```python
from build123d import *

# Parameters (mm, degrees)
PAD_DEPTH    = 9
SKETCH001_R  = 7
POCKET_DEPTH = 9
FILLET_R     = 50


with BuildPart() as part:
    # Sketch → Pad (new body)
    with BuildSketch(Plane.XY):
        Polygon((0, 94.860678), (0, 0), (0, -94.860678), (427.593604, -1000), (900, -1000), (900, 1000), (427.593604, 1000), align=None)
    extrude(amount=PAD_DEPTH)

    # Sketch001 (on DatumPlane) → Pocket (cut)
    with BuildSketch(Plane.XY.offset(9)):
        with Locations((328.804653, -388.309992)):
            Circle(SKETCH001_R)
        with Locations((116.672619, -176.177958)):
            Circle(SKETCH001_R)
    pocket = extrude(amount=-POCKET_DEPTH, mode=Mode.SUBTRACT)

    # Mirrored: Pocket across Sketch001 H_Axis
    add(pocket.mirror(Plane(origin=(0, 0, 9), x_dir=(0, 0, 1), z_dir=(0, 1, 0))), mode=Mode.SUBTRACT)

    # Fillet
    fillet_edges = [part.edges().sort_by_distance(p)[0] for p in [
        (0, 94.860678, 4.5),
        (0, -94.860678, 4.5),
        (427.593604, -1000, 4.5),
        (900, -1000, 4.5),
        (900, 1000, 4.5),
        (427.593604, 1000, 4.5),
    ]]
    fillet(fillet_edges, radius=FILLET_R)


with BuildPart() as part_1:
    # Fillet001Body placement: moved
    add(part.part.moved(Location((0, 0, 8))))


solid = part_1.part
```
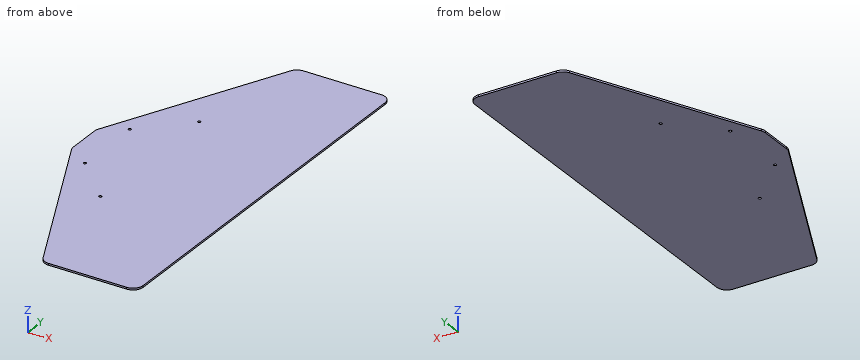
Could you check a few things on this model? Use its own coordinates, in mm. Round coordinates to 2 decimals unless told otherwise and drop trailing zeros. Loops run counter-clockwise (first coordinate to the right, second up) from the corner with the lowest first, then second, coordinate; pieces in that order, holes last. Notation, with made-up numbers: (28, 71) - (45, 71) arc R19 ccw to (45, 85) - close; hole circle Ø11 at (83.25, 12). An arc over 180 degrees is marked (long way). Answer in a Markdown table with one row per item. Add a question column.
(1) If we section it at C-C (y = 329.5): Please give me the cut outline in (x, z).
(2) I need wall thicknesses on line 1 along Y through (x, z) = (150, 15.25); line 2 along X through (y, z) = (-422, 9.75); line 3 along Y through (x, z) = (369, 15). Which ranges of each line are inside material? Lowest first, please.
(3) If we section it at B-B (x = 300): Please give me the cut outline in (y, z), plus the area to 3 significant figures.
(4) If we section it at A-A (z = 9.5): Please give me the cut outline in (x, y), plus the area to 3 significant figures.
(5) I'm going to push flat-ended pins straight in: pin 1 (12.5 mm diameter, centred on x = 328.8, y = -388.31, fed in from +Z); pin 2 (16 mm diameter, centred on x = 116.67, y = 176.18, fed in from -Z). Where does each tip first touch, or does it pass through?
Model answer:
| question | item | result |
|---|---|---|
| 1 | outline | (110.85, 8) - (900, 8) - (900, 17) - (110.85, 17) - close |
| 2 | line 1 | y = -412.38 to 412.38 |
| 2 | line 2 | x = 154.54 to 900 |
| 2 | line 3 | y = -875.97 to 875.97 |
| 3 | outline | (-729.91, 8) - (729.91, 8) - (729.91, 17) - (-729.91, 17) - close |
| 3 | area | 13,100 mm² |
| 4 | outline | (0, -83.64) arc R50 ccw to (4.79, -105) - (414.06, -971.36) arc R50 ccw to (459.27, -1000) - (850, -1000) arc R50 ccw to (900, -950) - (900, 950) arc R50 ccw to (850, 1000) - (459.27, 1000) arc R50 ccw to (414.06, 971.36) - (4.79, 105) arc R50 ccw to (0, 83.64) - close; hole circle Ø14 at (116.67, -176.18); hole circle Ø14 at (116.67, 176.18); hole circle Ø14 at (328.8, -388.31); hole circle Ø14 at (328.8, 388.31) |
| 4 | area | 1,410,000 mm² |
| 5 | pin 1 | passes through |
| 5 | pin 2 | stops at z = 8 |
